Autodesk Inventor part; units mm, degrees
ref_plane "YZ Plane" through (0, 0, 0) normal (1, 0, 0) x (0, 1, 0)
ref_plane "XZ Plane" through (0, 0, 0) normal (0, 1, 0) x (-1, 0, 0)
ref_plane "XY Plane" through (0, 0, 0) normal (0, 0, 1) x (1, 0, 0)
sketch "Sketch1" plane through (0, 0, 0) normal (0, 1, 0) x (-1, 0, 0)
  line L0 (0, 0) -> (152.4, 0)
  line L1 (152.4, 0) -> (152.4, -762)
  line L2 (0, -762) -> (0, 0)
  line L3 (152.4, -762) -> (0, -762) construction
  arc A0 (0, -762) -> (152.4, -762) centre (76.2, -936.5961) ccw
  line L4 (152.4, -590.1365) -> (152.4, -762) construction
  circle A1 centre (76.2, -936.5961) radius 60.325
  dimension "d1" = 762
  dimension "d5" = 381
  dimension "d6" = 120.65
  dimension "d11" = 762
extrude "Extrusion1" add sketch "Sketch1" along normal blind 12.7
fillet "Fillet1" radius 6.35 4 edges at (-76.2, 12.7, 0) (0, 12.7, -381) (-152.4, 12.7, -381) (-76.2, 12.7, -1127.0961)
sketch "Sketch2" plane through (0, 12.7, 0) normal (0, 1, 0) x (1, 0, 0)
  circle A0 centre (-76.2, 936.5961) radius 60.325 construction
  line L0 (-76.2, 936.5961) -> (-76.2, 876.2711) construction
  circle A1 centre (-76.2, 936.5961) radius 157.48 construction
  circle A2 centre (-233.68, 936.5961) radius 3.81
  circle A3 centre (-154.94, 800.2145) radius 3.81
  circle A4 centre (2.54, 800.2145) radius 3.81
  circle A5 centre (81.28, 936.5961) radius 3.81
  circle A6 centre (2.54, 1072.9778) radius 3.81
  circle A7 centre (-154.94, 1072.9778) radius 3.81
  point P0 (0, 0)
  dimension "d10" = 314.96
  dimension "d12" = 7.62
  dimension "d15" = 360
extrude "Extrusion2" cut sketch "Sketch2" against normal blind 12.7
sketch "Sketch3" plane through (0, 12.7, 0) normal (0, 1, 0) x (1, 0, 0)
  line L0 (0, 0) -> (-152.4, 0) construction
  line L1 (-76.2, 0) -> (-76.2, 12.7) construction
  line L2 (-76.2, 0) -> (-63.5, 0) construction
  line L3 (-12.7, 15.875) -> (-12.7, 60.325) construction
  line L4 (-15.875, 63.5) -> (-136.525, 63.5) construction
  line L5 (-139.7, 60.325) -> (-139.7, 15.875) construction
  line L6 (-136.525, 12.7) -> (-15.875, 12.7) construction
  circle A0 centre (-19.05, 57.15) radius 3.175
  circle A1 centre (-19.05, 57.15) radius 3.175
  circle A2 centre (-19.05, 19.05) radius 3.175
  circle A3 centre (-19.05, 19.05) radius 3.175
  circle A4 centre (-133.35, 57.15) radius 3.175
  circle A5 centre (-133.35, 57.15) radius 3.175
  circle A6 centre (-133.35, 19.05) radius 3.175
  arc A7 (-12.7, 60.325) -> (-15.875, 63.5) centre (-15.875, 60.325) ccw construction
  arc A8 (-15.875, 12.7) -> (-12.7, 15.875) centre (-15.875, 15.875) ccw construction
  arc A9 (-139.7, 15.875) -> (-136.525, 12.7) centre (-136.525, 15.875) ccw construction
  arc A10 (-136.525, 63.5) -> (-139.7, 60.325) centre (-136.525, 60.325) ccw construction
  line L7 (-76.2, 12.7) -> (-76.2, 63.5) construction
  line L8 (-76.2, 63.5) -> (-76.2, 584.2) construction
  line L9 (-139.7, 676.656) -> (-104.4, 676.656) construction
  line L10 (-139.7, 676.656) -> (-139.7, 587.375) construction
  line L11 (-136.525, 584.2) -> (-15.875, 584.2) construction
  line L12 (-12.7, 587.375) -> (-12.7, 676.656) construction
  line L13 (-12.7, 676.656) -> (-139.7, 676.656) construction
  arc A11 (-139.7, 587.375) -> (-136.525, 584.2) centre (-136.525, 587.375) ccw construction
  arc A12 (-15.875, 584.2) -> (-12.7, 587.375) centre (-15.875, 587.375) ccw construction
  circle A13 centre (-133.35, 590.55) radius 3.175
  circle A14 centre (-133.35, 590.55) radius 3.175
  circle A15 centre (-133.35, 628.65) radius 3.175
  circle A16 centre (-133.35, 628.65) radius 3.175
  circle A17 centre (-19.05, 590.55) radius 3.175
  circle A18 centre (-19.05, 590.55) radius 3.175
  circle A19 centre (-19.05, 628.65) radius 3.175
  circle A20 centre (-19.05, 628.65) radius 3.175
  line L14 (-76.2, 584.2) -> (-76.2, 676.656) construction
  point P0 (-12.7, 12.7)
  point P1 (-139.7, 635)
  dimension "d19" = 12.7
  dimension "d20" = 90
  dimension "d21" = 3.175
  dimension "d24" = 520.7
  dimension "d26" = 3.175
extrude "Extrusion3" cut sketch "Sketch3" against normal blind 12.7
properties part number "Arm Layer 1"
For this review, take the finished solid that the model builds, in its own axes (mm). Give positions to 0.01 mm unless a question says otherwise; leave off trailing zeros. Loops run counter-clockwise (first coordinate to the right, second up) from the corner with the lowest first, then second, coordinate; pieces in that order, holes last.
Item 1: Take a section at C-C, the plane y = 9.5. Give the number of separate pieces and of enclosed holes in the cut face, and give its area (3 significant figures).
Item 2: Take a section at B-B, the plane z = -73. State the section outline as (x, y) points, and give its area (3 significant figures).
Item 3: For line 1 along X through (y, z) = (4, -628.65) (3 decimals); line 2 along Z through (x, y) = (6, 1.75); line 3 along Z through (x, y) = (4, 5.75), list the stretches that pass through material, from the lowest coordinate up.
Item 4: Take a section at A-A, the plane x = -76.2. State the section outline as (y, z) points.
Item 5: Insertion check: pin 1 (1 mm diameter, centred on x = -4.5, z = -546, fed in from +Y); pin 2 (5 mm diameter, centred on x = -19.05, z = -57.15, fed in from +Y); pin 3 (5 mm diameter, centred on y = 2, z = -304, fed in from +X); pin 4 (1.5 mm diameter, centred on x = -48.5, y = 8, fed in from +Z). Each pin has a flat end and moves straight along its axis. Give the tip position at first contact, or say it passes through.
Calculated:
1. separate pieces: 1
1. enclosed holes: 15
1. area: 214,000 mm2
2. outline: (-152.4, 0) - (0, 0) - (0, 6.35) arc R6.35 ccw to (-6.35, 12.7) - (-146.05, 12.7) arc R6.35 ccw to (-152.4, 6.35) - close
2. area: 1,920 mm2
3. line 1: x = -152.4 to -136.525, -130.175 to -22.225, -15.875 to 0
3. line 2: z = -1108.45 to -1074.57, -1071.38 to -801.81, -798.62 to -764.74
3. line 3: z = -1109.39 to -1076.5, -1069.46 to -803.73, -796.7 to -763.8
4. outline: (0, -1127.1) - (6.35, -1127.1) arc R6.35 ccw to (12.7, -1120.75) - (12.7, -996.92) - (0, -996.92) - close; (0, -876.27) - (12.7, -876.27) - (12.7, -6.35) arc R6.35 ccw to (6.35, 0) - (0, 0) - close
5. pin 1: stops at y = 12.55
5. pin 2: passes through
5. pin 3: stops at x = 0
5. pin 4: stops at z = -0.06
